Autodesk Inventor part; units mm, degrees
ref_plane "YZ Plane" through (0, 0, 0) normal (1, 0, 0) x (0, 1, 0)
ref_plane "XZ Plane" through (0, 0, 0) normal (0, 1, 0) x (-1, 0, 0)
ref_plane "XY Plane" through (0, 0, 0) normal (0, 0, 1) x (1, 0, 0)
sketch "Sketch1" plane through (0, 0, 0) normal (1, 0, 0) x (0, 1, 0)
  line L0 (0, 0) -> (0, 597.7382)
  line L1 (0, 0) -> (3.175, 0)
  line L2 (3.175, 0) -> (3.175, 594.5632)
  line L3 (3.175, 594.5632) -> (9.906, 594.5632)
  line L4 (9.906, 594.5632) -> (15.756, 595.9828)
  line L5 (0, 597.7382) -> (9.5263, 597.7382)
  line L6 (9.5263, 597.7382) -> (12.7824, 598.5283)
  line L7 (41.2921, 902.0052) -> (15.756, 595.9828)
  line L8 (12.7824, 598.5283) -> (38.1281, 902.2692)
  line L9 (38.1281, 902.2692) -> (41.2921, 902.0052)
  line L10 (41.2921, 902.0052) -> (44.4671, 901.7403)
  line L11 (44.4671, 901.7403) -> (18.7409, 593.44)
  line L12 (18.7409, 593.44) -> (10.2857, 591.3882)
  line L13 (10.2857, 591.3882) -> (6.35, 591.3882)
  line L14 (6.35, 591.3882) -> (6.35, 574.5988)
  line L15 (6.35, 574.5988) -> (3.175, 574.5988)
  dimension "d0" = 594.5632
  dimension "d1" = 3.175
  dimension "d2" = 6.731
  dimension "d7" = 3.175
  dimension "d8" = 6.0198
  dimension "d9" = 166.36
  dimension "d10" = 3.175
  dimension "d11" = 108.41
  dimension "d12" = 3.175
  dimension "d13" = 307.086
  dimension "d16" = 3.175
  dimension "d18" = 3.175
  dimension "d20" = 307.1025
  dimension "d21" = 8.7006
  dimension "d22" = 3.175
  dimension "d23" = 3.175
  dimension "d24" = 3.9357
  dimension "d25" = 16.7894
extrude "Extrusion2" add sketch "Sketch1" along normal blind 1000.125 contours L2 L3 L4 L7 L10 L11 L12 L13 L14 L15
properties part number "First_Shingle_Over_Intake_Vent_With_Length_39.375_Inches"
Source: CAD feature listing. Evaluate the final solid. Frame: model axes, mm. A direction names the side the tool comes from. Round coordinates to 2 decimals unless told otherwise and drop trailing zeros. Loops run counter-clockwise (first coordinate to the right, second up) from the corner with the lowest first, then second, coordinate; pieces in that order, holes last.
1. Contact query for flat-ended pins moving along their axis: pin 1 (2 mm diameter, centred on x = 561, y = 7.5, fed in from -Z); pin 2 (3.5 mm diameter, centred on x = 427, y = 5.5, fed in from +Z); pin 3 (2 mm diameter, centred on x = 371.5, z = 615.5, fed in from +Y). Output: stop coordinate, or through.
2. Ray query, L1, parallel to Z at x = 703.5, y = 10.5; L2, parallel to Y at x = 511, z = 739; L3, parallel to Y at x = 233.5, z = 802. Return the intervals inside material, ascending.
3. Section query A-A on x = 741. Output: boundary loops of the cut face in (y, z) (3 decimals).
4. Access query for faces 1 (the flat face through (493, 6.35, 583)), 2 (the flat face through (0, 27, 715)). Directions: +Z, -Z, +X, -X, +Y, -Y. A direction counts if a zero-diameter tool reaches every point of the face in a straight line with its end or side. Return the directions, or none.
5. Section query B-B on y = 33. Output: boundary loops of the cut face in (x, z) (3 decimals).
6. Section query C-C on z = 708. Output: boundary loops of the cut face in (x, y) (3 decimals), and give its area (3 significant figures).
Answers below:
1. pin 1: stops at z = 591.39
1. pin 2: stops at z = 594.56
1. pin 3: stops at y = 20.67
2. L1: z = 591.44 to 594.71
2. L2: y = 27.69 to 30.89
2. L3: y = 32.95 to 36.14
3. outline: (3.175, 574.599) - (6.35, 574.599) - (6.35, 591.388) - (10.286, 591.388) - (18.741, 593.44) - (44.467, 901.74) - (41.292, 902.005) - (15.756, 595.983) - (9.906, 594.563) - (3.175, 594.563) - close
4. face 1: -Z, +X, -X, +Y
4. face 2: +Z, -Z, -X, +Y, -Y
5. outline: (0, 764.32) - (1000.125, 764.32) - (1000.125, 802.633) - (0, 802.633) - close
6. outline: (0, 25.103) - (1000.125, 25.103) - (1000.125, 28.3) - (0, 28.3) - close
6. area: 3,200 mm2
